Can you work these out from the model? Positions are in its coordinate system, mm. A direction names the side the tool comes from. Give positions to 0.01 mm unless a question says otherwise; leave off trailing zeros. Write each loop counter-clockwise with the first axis right and the second up, starting at its lowest first coordinate (ties: lowest second). Pieces come first, ordered by that corner, then holes. Notation, with made-up numbers: (-10, 68.5) - (3, 68.5) arc R18 cw to (3, 102.5) - close; hole circle Ø8 at (-26, -12). An arc over 180 degrees is marked (long way). Return JSON: item names as keys, results as strings. Group by question number.
from build123d import *

# Parameters (mm, degrees)
F2_SIZE2 = 0.6516126864
F2_SIZE  = 0.5
F3_R     = 1
F4_R     = 12
F5_DEPTH = 25


with BuildPart() as f1:
    # F0 (on Front) → F1 (revolve)
    with BuildSketch(Plane.XZ):
        Polygon((-27.3038475773, 4), (0, 4), (0, 5), (-8, 5), (-16.5, 8), (-16.5, 12), (-24.5, 12), (-24.5, 8), (-38.5, 8), (-38.5, 7), align=None)
    revolve(axis=Axis((0.1931033472, 0, 0), (1, 0, 0)))

    # F2
    f2_edges = [f1.edges().sort_by_distance(p)[0] for p in [
        (0, 0, -5),
    ]]
    f2_side = f1.faces().sort_by_distance((-4, 0, -5))[0]
    chamfer(f2_edges, length=F2_SIZE, length2=F2_SIZE2, reference=f2_side)

    # F3
    f3_edges = [f1.edges().sort_by_distance(p)[0] for p in [
        (-16.5, 0, -8),
        (-8, 0, -5),
    ]]
    fillet(f3_edges, radius=F3_R)

    # F4 (on face) → F5 (cut)
    with BuildSketch(Plane(origin=(-24.5, 0, 0), x_dir=(0, -1, 0), z_dir=(-1, 0, 0))):
        Circle(F4_R)
        Polygon((-9.5, -5.4848275573), (-9.5, 5.4848275573), (0, 10.9696551146), (9.5, 5.4848275573), (9.5, -5.4848275573), (0, -10.9696551146), align=None, mode=Mode.SUBTRACT)
    extrude(amount=-F5_DEPTH, mode=Mode.SUBTRACT)

    # F6 (on Front) → F7 (revolve, cut)
    with BuildSketch(Plane.XZ):
        Polygon((-24.5, 13.6036825632), (-24.5, 10.9696551146), (-24.5, 9), (-23.266446975, 13.6036825632), align=None)
        Polygon((-17.733553025, 13.6036825632), (-16.5, 9), (-16.5, 10.9696551146), (-16.5, 13.6036825632), align=None)
    revolve(axis=Axis((5.1041673869, 0, 0), (1, 0, 0)), mode=Mode.SUBTRACT)


solid = f1.part
1) On a 3-axis mill with a long thin cutter (end or side, diameter ignored), from which of +Z, -Z, +X, -X, +Y, -Y can I reach the whole of each face in a straight line? I mean faces 1 (the face through (-4, -4, 3)), 2 (the face through (-20.6, -4.8, -8.2)), 3 (the face through (-31.6, 7.81, -1.73)). Say none if no direction works.
2) Imagine slicing it at A-A, the plane x = -6. Write out the boundary of the cut face in (y, z).
3) We'd pull the mould along Y, two halves only. Please class faces 4 (the face through (-13.461, 3.905, -0.867)), 5 (the face through (-20.554, 4.684, -8.266)), 6 (the face through (-20.554, -4.684, 8.266)): pulls with the +Y half, pulls with the -Y half, needs draft (parallel to the pull), parting line crosses it, or undercut.
4) Will these pins go through, and if not, where does the flat tip stop? pin 1 Ø2 at (y, z) = (-5, 2.5) entering from +X; pin 2 Ø9 at (y, z) = (-3, -2.5) entering from +X; pin 3 Ø1.5 at (x, y) = (-5, 0.5) entering from +Z; pin 4 Ø6 at (x, y) = (-30, -5.5) entering from +Z.
5) Imagine slicing it at B-B, the plane x = -31. Write out the boundary of the cut face in (y, z).
6) I need wall thicknesses on line 1 along Z through (x, y) = (-6, 0); line 2 along Z through (x, y) = (-21, 0); line 3 along Y through (x, z) = (-34.5, -1.25). Which ranges of each line are inside material? Lowest first, please.
Resolved:
{
 "1": {"face 1": "+X", "face 2": "-Z, +X, -X, -Y", "face 3": "-X"},
 "2": {"outline": "circle Ø10 at (0, 0); hole circle Ø8 at (0, 0)"},
 "3": {"face 4": "undercut", "face 5": "pulls with the +Y half", "face 6": "pulls with the -Y half"},
 "4": {"pin 1": "x = -0.19", "pin 2": "x = 0", "pin 3": "z = 5", "pin 4": "z = 7.6"},
 "5": {"outline": "circle Ø16 at (0, 0); hole circle Ø9.98 at (0, 0)"},
 "6": {"line 1": "-5 to -4, 4 to 5", "line 2": "-10.97 to -4, 4 to 10.97", "line 3": "-7.9 to -5.79, 5.79 to 7.9"}
}
